from build123d import *

# Parameters (mm, degrees)
ESQUISSE1_W             = 215
ESQUISSE1_H             = 85.5
ESQUISSE1_W_2           = 40
ESQUISSE1_H_2           = 5
BOSS_EXTRU_1_DEPTH      = 2
CONG_1_R                = 6
CONG_2_R                = 20
CONG_3_R                = 2.5
ENL_V_MAT_EXTRU_1_REACH = 233.386


with BuildPart() as part:
    # Esquisse1 → Boss.-Extru.1 (new body)
    with BuildSketch(Plane.XY):
        with Locations((107.5, 42.75)):
            Rectangle(ESQUISSE1_W, ESQUISSE1_H)
        with Locations((155, 7.5)):
            Rectangle(ESQUISSE1_W_2, ESQUISSE1_H_2, mode=Mode.SUBTRACT)
        with Locations((155, 78)):
            Rectangle(ESQUISSE1_W_2, ESQUISSE1_H_2, mode=Mode.SUBTRACT)
        with Locations((40, 7.5)):
            Rectangle(ESQUISSE1_W_2, ESQUISSE1_H_2, mode=Mode.SUBTRACT)
        with Locations((40, 78)):
            Rectangle(ESQUISSE1_W_2, ESQUISSE1_H_2, mode=Mode.SUBTRACT)
    extrude(amount=BOSS_EXTRU_1_DEPTH)

    # Congé1
    cong_1_edges = [part.edges().sort_by_distance(p)[0] for p in [
        (215, 85.5, 1),
        (215, 0, 1),
    ]]
    fillet(cong_1_edges, radius=CONG_1_R)

    # Congé2
    cong_2_edges = [part.edges().sort_by_distance(p)[0] for p in [
        (0, 85.5, 1),
        (0, 0, 1),
    ]]
    fillet(cong_2_edges, radius=CONG_2_R)

    # Congé3
    cong_3_edges = [part.edges().sort_by_distance(p)[0] for p in [
        (20, 80.5, 1),
        (20, 75.5, 1),
        (60, 75.5, 1),
        (60, 80.5, 1),
        (60, 10, 1),
        (60, 5, 1),
        (20, 5, 1),
        (20, 10, 1),
        (135, 10, 1),
        (135, 5, 1),
        (175, 10, 1),
        (175, 5, 1),
        (135, 80.5, 1),
        (135, 75.5, 1),
        (175, 75.5, 1),
        (175, 80.5, 1),
    ]]
    fillet(cong_3_edges, radius=CONG_3_R - 0.0001)  # a hair under: the kernel refuses the full size

    # Esquisse2 → Enlèv. mat.-Extru.1 (cut, up to next)
    with BuildSketch(Plane(origin=(0, 0, 0), x_dir=(-1, 0, 0), z_dir=(0, 0, -1)), mode=Mode.PRIVATE) as enl_v_mat_extru_1_sk1:
        Polygon((-87.246997481, 38.721191603), (-88.332391174, 53.664112074), (-69.444138278, 55.03607886), (-68.358744585, 40.093158389), align=None)
    enl_v_mat_extru_1_tool1 = extrude(enl_v_mat_extru_1_sk1.sketch, amount=-ENL_V_MAT_EXTRU_1_REACH, mode=Mode.PRIVATE) & part.part
    # Esquisse2 → Enlèv. mat.-Extru.1 (cut, up to next)
    with BuildSketch(Plane(origin=(0, 0, 0), x_dir=(-1, 0, 0), z_dir=(0, 0, -1)), mode=Mode.PRIVATE) as enl_v_mat_extru_1_sk2:
        Polygon((-118.903285372, 35.932207835), (-120.210621513, 50.875128306), (-105.267701042, 52.182464448), (-103.9603649, 37.239543976), align=None)
    enl_v_mat_extru_1_tool2 = extrude(enl_v_mat_extru_1_sk2.sketch, amount=-ENL_V_MAT_EXTRU_1_REACH, mode=Mode.PRIVATE) & part.part
    add(enl_v_mat_extru_1_tool1.solids().sort_by_distance((78.345568, 46.878635, 0))[0], mode=Mode.SUBTRACT)
    add(enl_v_mat_extru_1_tool2.solids().sort_by_distance((112.085493, 44.057336, 0))[0], mode=Mode.SUBTRACT)


solid = part.part
Here's how the part is built. I have some questions about the finished solid (model axes, mm). Round coordinates to 2 decimals unless told otherwise and drop trailing zeros. Order: outer loops, then holes, each group sorted by start corner. A loop starts at its lowest first (then second) coordinate and runs counter-clockwise, first axis right, second up. Notation, with made-up numbers: (-32.5, 11.25) -> (-10.5, 11.25) arc R18 ccw to (-10.5, 37.25) -> close; hole circle Ø7 at (14.25, 55). An arc over 180 degrees is marked (long way). Use CSV: the item, a comma, the result in double quotes.
1. I want a section at A-A on x = 141. List the corners of the cut face in (y, z) for me, and give its area (3 significant figures).
Recorded:
outline,"(0, 0) -> (5, 0) -> (5, 2) -> (0, 2) -> close; (10, 0) -> (75.5, 0) -> (75.5, 2) -> (10, 2) -> close; (80.5, 0) -> (85.5, 0) -> (85.5, 2) -> (80.5, 2) -> close"
area,"151 mm2"
2. I need wall thicknesses on line 1 along Y through (x, z) = (170, 0.95); line 2 along Y through (x, z) = (173, 1); line 3 along X through (y, z) = (49, 0.95). Which ranges of each line are inside material? Lowest first, please.
Recorded:
line 1,"y = 0 to 5, 10 to 75.5, 80.5 to 85.5"
line 2,"y = 0 to 5.05, 9.95 to 75.55, 80.45 to 85.5"
line 3,"x = 0 to 69.01, 87.99 to 104.99, 120.05 to 215"
3. I want a section at B-B on z = 1.45. Give the number of separate pieces and of enclosed holes in the cut face, and give its area (3 significant figures).
Recorded:
separate pieces,"1"
enclosed holes,"6"
area,"16,900 mm2"
